```python
from build123d import *

# Parameters (mm, degrees)
F1_DEPTH = 4
F2_R     = 2
F2_R_2   = 3.5
F3_DEPTH = 25
F4_R     = 4.99999


# Not quite as in the source:
# - a fillet or chamfer is up to 0.001 mm smaller than in the source, because OpenCascade refuses the exact size


with BuildPart() as f1:
    # F0 (on Top) → F1 (new body)
    with BuildSketch(Plane.XY):
        Polygon((-5, 65), (-5, 0), (-35, 0), (-35, -14), (35, -14), (35, 0), (5, 0), (5, 65), align=None)
    extrude(amount=F1_DEPTH)

    # F2 (on face) → F3 (cut)
    with BuildSketch(Plane.XY.offset(4)):
        with Locations((-30, -7)):
            Circle(F2_R)
        with Locations((30, -7)):
            Circle(F2_R)
        with Locations((0, -7)):
            Circle(F2_R_2)
        with Locations((0, 61)):
            Circle(F2_R)
    extrude(amount=-F3_DEPTH, mode=Mode.SUBTRACT)

    # F4 (radius 5 in the source; OpenCascade refuses exactly that, so slightly less here)
    f4_edges = [f1.edges().sort_by_distance(p)[0] for p in [
        (-35, -14, 2),
        (-35, 0, 2),
        (35, -14, 2),
        (35, 0, 2),
        (5, 65, 2),
        (-5, 65, 2),
    ]]
    fillet(f4_edges, radius=F4_R)


solid = f1.part
```
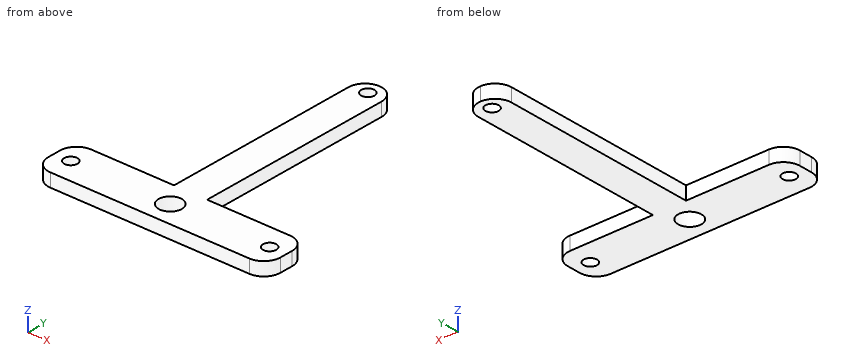
Input: part model. Units: mm. Frame: model coordinates. Give positions to 0.01 mm unless a question says otherwise; leave off trailing zeros. Order: outer loops, then holes, each group sorted by start corner. A loop starts at its lowest first (then second) coordinate and runs counter-clockwise, first axis right, second up. Notation, with made-up numbers: M 2.25,30 L 7.25,30 A23 cw 7.25,50 Z; hole C -1,85.25 d3. An arc over 180 degrees is marked long. One line per question, with ' | ' between items.
1) Section A-A on z = 3.3. State how many separate pieces and enclosed holes the cut face has, and give its area (3 significant figures).
Filled in:
separate pieces: 1 | enclosed holes: 4 | area: 1,520 mm2
2) Ray query, L1, parallel to Y at x = 0, z = 2.7; L2, parallel to Y at x = -1, z = 0.6; L3, parallel to X at y = 30, z = 1.8. Return the intervals inside material, ascending.
Filled in:
L1: y = -14 to -10.5, -3.5 to 59, 63 to 65 | L2: y = -14 to -10.35, -3.65 to 59.27, 62.73 to 64.9 | L3: x = -5 to 5
3) Section B-B on y = 61. Output: boundary loops of the cut face in (x, z), and give its area (3 significant figures).
Filled in:
outline: M -4.9,0 L -2,0 L -2,4 L -4.9,4 Z; M 2,0 L 4.9,0 L 4.9,4 L 2,4 Z | area: 23.2 mm2
4) Section C-C on x = -24. Output: boundary loops of the cut face in (y, z).
Filled in:
outline: M -14,0 L 0,0 L 0,4 L -14,4 Z
5) Section D-D on y = 6. Output: boundary loops of the cut face in (x, z), and give its area (3 significant figures).
Filled in:
outline: M -5,0 L 5,0 L 5,4 L -5,4 Z | area: 40.0 mm2
6) Contact query for flat-ended pins moving along their axis: P1, Ø1.2, axis at y = 21.5, z = 2, coming from the +X side; P2, Ø6.5, axis at x = 0, y = -7, coming from the +Z side; P3, Ø1.5, axis at x = -10.5, z = 3.5, coming from the +Y side. Output: stop coordinate, or through.
Filled in:
P1: stops at x = 5 | P2: passes through | P3: stops at y = 0
